```python
from build123d import *

# Parameters (mm, degrees)
F0_R     = 6.25
F1_DEPTH = 7.5
F2_DEPTH = 2.5
F3_R     = 1
F4_SIZE  = 1


with BuildPart() as f1:
    # F0 (on Top) → F1 (new body)
    with BuildSketch(Plane.XY):
        with BuildLine():
            Line((-15.2574911714, 10), (-40.2574911714, 10))
            ThreePointArc((-40.2574911714, 10), (-50.2574911714, 0), (-40.2574911714, -10))
            Line((-40.2574911714, -10), (-20.2574911714, -10))
            ThreePointArc((-20.2574911714, -10), (-16.7219572654, -11.4644660941), (-15.2574911714, -15))
            Line((-15.2574911714, -15), (-15.2574911714, -30.0000000031))
            Line((-15.2574911714, -30.0000000031), (4.7425088286, -30.0000000031))
            Line((4.7425088286, -30.0000000031), (4.7425088286, -10))
            ThreePointArc((4.7425088286, -10), (-1.1153555476, 4.1421356237), (-15.2574911714, 10))
        make_face()
        with Locations((-40.2574911714, 0)):
            Circle(F0_R, mode=Mode.SUBTRACT)
    extrude(amount=-F1_DEPTH)

    # F0 (on Top) → F2 (join)
    with BuildSketch(Plane.XY):
        with BuildLine():
            Line((13.7208224833, -30.0000000031), (4.7425088286, -30.0000000031))
            Line((4.7425088286, -30.0000000031), (-15.2574911714, -30.0000000031))
            Line((-15.2574911714, -30.0000000031), (-26.2791775167, -30.0000000031))
            Line((-26.2791775167, -30.0000000031), (-26.2791775167, -45.0000000031))
            ThreePointArc((-26.2791775167, -45.0000000031), (-24.8147114226, -48.535533909), (-21.2791775167, -50.0000000031))
            Line((-21.2791775167, -50.0000000031), (8.7208224833, -50.0000000031))
            ThreePointArc((8.7208224833, -50.0000000031), (12.2563563892, -48.535533909), (13.7208224833, -45.0000000031))
            Line((13.7208224833, -45.0000000031), (13.7208224833, -30.0000000031))
        make_face()
    extrude(amount=-F2_DEPTH)

    # F3
    f3_edges = [f1.edges().sort_by_distance(p)[0] for p in [
        (-46.507491, 0, -7.5),
        (-27.757491, 10, -7.5),
        (-50.257491, 0, -7.5),
        (-30.257491, -10, -7.5),
        (-16.721957, -11.464466, -7.5),
        (-15.257491, -22.5, -7.5),
        (-5.257491, -30, -7.5),
        (4.742509, -20, -7.5),
        (-1.115356, 4.142136, -7.5),
        (-5.257491, -30, -2.5),
    ]]
    fillet(f3_edges, radius=F3_R)

    # F4
    f4_edges = [f1.edges().sort_by_distance(p)[0] for p in [
        (-27.757491, 10, 0),
        (-50.257491, 0, 0),
        (-30.257491, -10, 0),
        (-16.721957, -11.464466, 0),
        (-15.257491, -22.5, 0),
        (-20.768334, -30, 0),
        (-26.279178, -37.5, 0),
        (-24.814711, -48.535534, 0),
        (-6.279178, -50, 0),
        (12.256356, -48.535534, 0),
        (13.720822, -37.5, 0),
        (9.231666, -30, 0),
        (4.742509, -20, 0),
        (-1.115356, 4.142136, 0),
        (-46.507491, 0, 0),
    ]]
    chamfer(f4_edges, length=F4_SIZE)


solid = f1.part
```
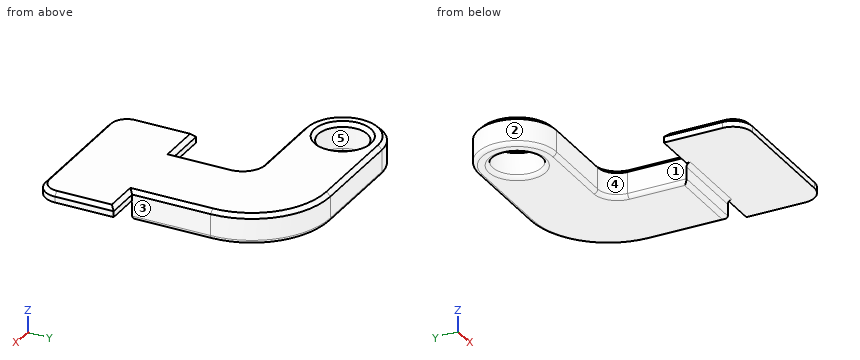
Check sheet for the modelled part. Datum: model origin and axes. Units: mm. Face numbers are marked on the shaded views. A direction names the side the tool comes from. Round coordinates to 2 decimals unless told otherwise and drop trailing zeros. Loops run counter-clockwise (first coordinate to the right, second up) from the corner with the lowest first, then second, coordinate; pieces in that order, holes last. Notation, with made-up numbers: (-29, -35) - (-2, -35) arc R36 ccw to (-2, 2) - close; hole circle Ø5 at (-4, -38). An arc over 180 degrees is marked (long way). Write item = value, one per line. Start each with the question number.
Q1. Access from +Z, -Z, +X, -X, +Y, -Y to the whole of each face (thin tool, end or side, straight path). Record for the marked faces 4 and 5.
Q2. Section check B-B (x = 6). Record the boundary of the cut face in (y, z), plus the area to 3 significant figures.
Q3. Thickness scan on L1, parallel to X at y = -16, z = -5.25; L2, parallel to Y at x = -33, z = -4.5; L3, parallel to Y at x = -18.5, z = -1. Record the ranges inside material, lowest first.
Q4. Depth check by flat-ended pin: P1, Ø1, axis at x = -28, z = -6.5, coming from the -Y side; P2, Ø0.8, axis at x = 10.5, z = -2, coming from the +Y side; P3, Ø1.5, axis at x = 6.5, y = -36, coming from the -Z side. Enter the tip coordinate at first touch or a pass-through.
Q5. Section check C-C (y = -33.5). Record the boundary of the cut face in (x, z).
Q6. Section check A-A (y = -25.5). Record the boundary of the cut face in (x, z).
Q7. Release check for a two-part mould opening along Y. For the marked faces 1, 2 and 3 record: pulls with the +Y half, pulls with the -Y half, needs draft (parallel to the pull), parting line crosses it, or undercut.
Derived:
q1.face_4 = +Z, -Z, -X
q1.face_5 = +Z, -Z
q2.outline = (-50, -2.5) - (-30, -2.5) - (-30, -1) - (-31, 0) - (-49, 0) - (-50, -1) - close
q2.area = 49.0 mm^2
q3.L1 = -15.26 to 4.74
q3.L2 = -10 to 10
q3.L3 = -50 to -30, -10.32 to 10
q4.P1 = -10
q4.P2 = -30
q4.P3 = -2.5
q5.outline = (-26.28, -2.5) - (13.72, -2.5) - (13.72, -1) - (12.72, 0) - (-25.28, 0) - (-26.28, -1) - close
q6.outline = (-15.26, -6.5) arc R1 ccw to (-14.26, -7.5) - (3.74, -7.5) arc R1 ccw to (4.74, -6.5) - (4.74, -1) - (3.74, 0) - (-14.26, 0) - (-15.26, -1) - close
q7.face_1 = undercut
q7.face_2 = parting line crosses it
q7.face_3 = needs draft
